```python
from build123d import *

# Parameters (mm, degrees)
SKETCH_1_R      = 3.4
SKETCH_1_W      = 10.3
SKETCH_1_H      = 10.3
EXTRUDE_1_DEPTH = 100


with BuildPart() as part:
    # 草图1 → 凸台-拉伸1 (new body)
    with BuildSketch(Plane.XY):
        with BuildLine():
            Line((-22.463172707, 9.357012623), (-25.363172707, 9.357012623))
            Line((-25.363172707, 9.357012623), (-25.363172707, 17.757012623))
            Line((-25.363172707, 17.757012623), (-22.963172707, 17.757012623))
            ThreePointArc((-22.963172707, 17.757012623), (-22.609619316, 17.903459232), (-22.463172707, 18.257012623))
            Line((-22.463172707, 18.257012623), (-22.463172707, 20.257012623))
            ThreePointArc((-22.463172707, 20.257012623), (-22.609619316, 20.610566013), (-22.963172707, 20.757012623))
            Line((-22.963172707, 20.757012623), (-37.863172707, 20.757012623))
            ThreePointArc((-37.863172707, 20.757012623), (-38.216726098, 20.610566013), (-38.363172707, 20.257012623))
            Line((-38.363172707, 20.257012623), (-38.363172707, 5.357012623))
            ThreePointArc((-38.363172707, 5.357012623), (-38.216726098, 5.003459232), (-37.863172707, 4.857012623))
            Line((-37.863172707, 4.857012623), (-35.863172707, 4.857012623))
            ThreePointArc((-35.863172707, 4.857012623), (-35.509619316, 5.003459232), (-35.363172707, 5.357012623))
            Line((-35.363172707, 5.357012623), (-35.363172707, 7.757012623))
            Line((-35.363172707, 7.757012623), (-26.963172707, 7.757012623))
            Line((-26.963172707, 7.757012623), (-26.963172707, 4.857012623))
            Line((-26.963172707, 4.857012623), (-25.420279488, 6.399905842))
            Line((-25.420279488, 6.399905842), (-23.217718457, 4.19734481))
            ThreePointArc((-23.217718457, 4.19734481), (-24.313172707, 0.757012623), (-23.217718457, -2.683319565))
            Line((-23.217718457, -2.683319565), (-25.420279488, -4.885880596))
            Line((-25.420279488, -4.885880596), (-26.963172707, -3.342987377))
            Line((-26.963172707, -3.342987377), (-26.963172707, -6.242987377))
            Line((-26.963172707, -6.242987377), (-35.363172707, -6.242987377))
            Line((-35.363172707, -6.242987377), (-35.363172707, -3.842987377))
            ThreePointArc((-35.363172707, -3.842987377), (-35.509619316, -3.489433987), (-35.863172707, -3.342987377))
            Line((-35.863172707, -3.342987377), (-37.863172707, -3.342987377))
            ThreePointArc((-37.863172707, -3.342987377), (-38.216726098, -3.489433987), (-38.363172707, -3.842987377))
            Line((-38.363172707, -3.842987377), (-38.363172707, -18.742987377))
            ThreePointArc((-38.363172707, -18.742987377), (-38.216726098, -19.096540768), (-37.863172707, -19.242987377))
            Line((-37.863172707, -19.242987377), (-22.963172707, -19.242987377))
            ThreePointArc((-22.963172707, -19.242987377), (-22.609619316, -19.096540768), (-22.463172707, -18.742987377))
            Line((-22.463172707, -18.742987377), (-22.463172707, -16.742987377))
            ThreePointArc((-22.463172707, -16.742987377), (-22.609619316, -16.389433987), (-22.963172707, -16.242987377))
            Line((-22.963172707, -16.242987377), (-25.363172707, -16.242987377))
            Line((-25.363172707, -16.242987377), (-25.363172707, -7.842987377))
            Line((-25.363172707, -7.842987377), (-22.463172707, -7.842987377))
            Line((-22.463172707, -7.842987377), (-24.006065926, -6.300094158))
            Line((-24.006065926, -6.300094158), (-21.803504895, -4.097533127))
            ThreePointArc((-21.803504895, -4.097533127), (-18.363172707, -5.192987377), (-14.922840519, -4.097533127))
            Line((-14.922840519, -4.097533127), (-12.720279488, -6.300094158))
            Line((-12.720279488, -6.300094158), (-14.263172707, -7.842987377))
            Line((-14.263172707, -7.842987377), (-11.363172707, -7.842987377))
            Line((-11.363172707, -7.842987377), (-11.363172707, -16.242987377))
            Line((-11.363172707, -16.242987377), (-13.763172707, -16.242987377))
            ThreePointArc((-13.763172707, -16.242987377), (-14.116726098, -16.389433987), (-14.263172707, -16.742987377))
            Line((-14.263172707, -16.742987377), (-14.263172707, -18.742987377))
            ThreePointArc((-14.263172707, -18.742987377), (-14.116726098, -19.096540768), (-13.763172707, -19.242987377))
            Line((-13.763172707, -19.242987377), (1.136827293, -19.242987377))
            Line((1.136827293, -19.242987377), (2.136827293, -19.242987377))
            Line((2.136827293, -19.242987377), (17.036827293, -19.242987377))
            ThreePointArc((17.036827293, -19.242987377), (17.390380684, -19.096540768), (17.536827293, -18.742987377))
            Line((17.536827293, -18.742987377), (17.536827293, -16.742987377))
            ThreePointArc((17.536827293, -16.742987377), (17.390380684, -16.389433987), (17.036827293, -16.242987377))
            Line((17.036827293, -16.242987377), (14.636827293, -16.242987377))
            Line((14.636827293, -16.242987377), (14.636827293, -7.842987377))
            Line((14.636827293, -7.842987377), (17.536827293, -7.842987377))
            Line((17.536827293, -7.842987377), (15.993934074, -6.300094158))
            Line((15.993934074, -6.300094158), (18.196495105, -4.097533127))
            ThreePointArc((18.196495105, -4.097533127), (21.636827293, -5.192987377), (25.077159481, -4.097533127))
            Line((25.077159481, -4.097533127), (27.279720512, -6.300094158))
            Line((27.279720512, -6.300094158), (25.736827293, -7.842987377))
            Line((25.736827293, -7.842987377), (28.636827293, -7.842987377))
            Line((28.636827293, -7.842987377), (28.636827293, -16.242987377))
            Line((28.636827293, -16.242987377), (26.236827293, -16.242987377))
            ThreePointArc((26.236827293, -16.242987377), (25.883273902, -16.389433987), (25.736827293, -16.742987377))
            Line((25.736827293, -16.742987377), (25.736827293, -18.742987377))
            ThreePointArc((25.736827293, -18.742987377), (25.883273902, -19.096540768), (26.236827293, -19.242987377))
            Line((26.236827293, -19.242987377), (41.136827293, -19.242987377))
            ThreePointArc((41.136827293, -19.242987377), (41.490380684, -19.096540768), (41.636827293, -18.742987377))
            Line((41.636827293, -18.742987377), (41.636827293, -3.842987377))
            ThreePointArc((41.636827293, -3.842987377), (41.490380684, -3.489433987), (41.136827293, -3.342987377))
            Line((41.136827293, -3.342987377), (39.136827293, -3.342987377))
            ThreePointArc((39.136827293, -3.342987377), (38.783273902, -3.489433987), (38.636827293, -3.842987377))
            Line((38.636827293, -3.842987377), (38.636827293, -6.242987377))
            Line((38.636827293, -6.242987377), (30.236827293, -6.242987377))
            Line((30.236827293, -6.242987377), (30.236827293, -3.342987377))
            Line((30.236827293, -3.342987377), (28.693934074, -4.885880596))
            Line((28.693934074, -4.885880596), (26.491373043, -2.683319565))
            ThreePointArc((26.491373043, -2.683319565), (27.586827293, 0.757012623), (26.491373043, 4.19734481))
            Line((26.491373043, 4.19734481), (28.693934074, 6.399905842))
            Line((28.693934074, 6.399905842), (30.236827293, 4.857012623))
            Line((30.236827293, 4.857012623), (30.236827293, 7.757012623))
            Line((30.236827293, 7.757012623), (38.636827293, 7.757012623))
            Line((38.636827293, 7.757012623), (38.636827293, 5.357012623))
            ThreePointArc((38.636827293, 5.357012623), (38.783273902, 5.003459232), (39.136827293, 4.857012623))
            Line((39.136827293, 4.857012623), (41.136827293, 4.857012623))
            ThreePointArc((41.136827293, 4.857012623), (41.490380684, 5.003459232), (41.636827293, 5.357012623))
            Line((41.636827293, 5.357012623), (41.636827293, 20.257012623))
            ThreePointArc((41.636827293, 20.257012623), (41.490380684, 20.610566013), (41.136827293, 20.757012623))
            Line((41.136827293, 20.757012623), (26.236827293, 20.757012623))
            ThreePointArc((26.236827293, 20.757012623), (25.883273902, 20.610566013), (25.736827293, 20.257012623))
            Line((25.736827293, 20.257012623), (25.736827293, 18.257012623))
            ThreePointArc((25.736827293, 18.257012623), (25.883273902, 17.903459232), (26.236827293, 17.757012623))
            Line((26.236827293, 17.757012623), (28.636827293, 17.757012623))
            Line((28.636827293, 17.757012623), (28.636827293, 9.357012623))
            Line((28.636827293, 9.357012623), (25.736827293, 9.357012623))
            Line((25.736827293, 9.357012623), (27.279720512, 7.814119404))
            Line((27.279720512, 7.814119404), (25.077159481, 5.611558373))
            ThreePointArc((25.077159481, 5.611558373), (21.636827293, 6.707012623), (18.196495105, 5.611558373))
            Line((18.196495105, 5.611558373), (15.993934074, 7.814119404))
            Line((15.993934074, 7.814119404), (17.536827293, 9.357012623))
            Line((17.536827293, 9.357012623), (14.636827293, 9.357012623))
            Line((14.636827293, 9.357012623), (14.636827293, 17.757012623))
            Line((14.636827293, 17.757012623), (17.036827293, 17.757012623))
            ThreePointArc((17.036827293, 17.757012623), (17.390380684, 17.903459232), (17.536827293, 18.257012623))
            Line((17.536827293, 18.257012623), (17.536827293, 20.257012623))
            ThreePointArc((17.536827293, 20.257012623), (17.390380684, 20.610566013), (17.036827293, 20.757012623))
            Line((17.036827293, 20.757012623), (2.136827293, 20.757012623))
            Line((2.136827293, 20.757012623), (1.136827293, 20.757012623))
            Line((1.136827293, 20.757012623), (-13.763172707, 20.757012623))
            ThreePointArc((-13.763172707, 20.757012623), (-14.116726098, 20.610566013), (-14.263172707, 20.257012623))
            Line((-14.263172707, 20.257012623), (-14.263172707, 18.257012623))
            ThreePointArc((-14.263172707, 18.257012623), (-14.116726098, 17.903459232), (-13.763172707, 17.757012623))
            Line((-13.763172707, 17.757012623), (-11.363172707, 17.757012623))
            Line((-11.363172707, 17.757012623), (-11.363172707, 9.357012623))
            Line((-11.363172707, 9.357012623), (-14.263172707, 9.357012623))
            Line((-14.263172707, 9.357012623), (-12.720279488, 7.814119404))
            Line((-12.720279488, 7.814119404), (-14.922840519, 5.611558373))
            ThreePointArc((-14.922840519, 5.611558373), (-18.363172707, 6.707012623), (-21.803504895, 5.611558373))
            Line((-21.803504895, 5.611558373), (-24.006065926, 7.814119404))
            Line((-24.006065926, 7.814119404), (-22.463172707, 9.357012623))
        make_face()
        with Locations((-18.363172707, 0.757012623)):
            Circle(SKETCH_1_R, mode=Mode.SUBTRACT)
        with Locations((21.636827293, 0.757012623)):
            Circle(SKETCH_1_R, mode=Mode.SUBTRACT)
        with Locations((-31.513172707, 13.907012623)):
            Rectangle(SKETCH_1_W, SKETCH_1_H, mode=Mode.SUBTRACT)
        with BuildLine():
            Line((-9.363172707, 17.757012623), (-9.363172707, 8.34279906))
            Line((-9.363172707, 8.34279906), (-13.508626957, 4.19734481))
            ThreePointArc((-13.508626957, 4.19734481), (-12.413172707, 0.757012623), (-13.508626957, -2.683319565))
            Line((-13.508626957, -2.683319565), (-9.363172707, -6.828773815))
            Line((-9.363172707, -6.828773815), (-9.363172707, -16.242987377))
            ThreePointArc((-9.363172707, -16.242987377), (-9.070279488, -16.950094158), (-8.363172707, -17.242987377))
            Line((-8.363172707, -17.242987377), (11.636827293, -17.242987377))
            ThreePointArc((11.636827293, -17.242987377), (12.343934074, -16.950094158), (12.636827293, -16.242987377))
            Line((12.636827293, -16.242987377), (12.636827293, -6.828773815))
            Line((12.636827293, -6.828773815), (16.782281543, -2.683319565))
            ThreePointArc((16.782281543, -2.683319565), (15.686827293, 0.757012623), (16.782281543, 4.19734481))
            Line((16.782281543, 4.19734481), (12.636827293, 8.34279906))
            Line((12.636827293, 8.34279906), (12.636827293, 17.757012623))
            ThreePointArc((12.636827293, 17.757012623), (12.343934074, 18.464119404), (11.636827293, 18.757012623))
            Line((11.636827293, 18.757012623), (-8.363172707, 18.757012623))
            ThreePointArc((-8.363172707, 18.757012623), (-9.070279488, 18.464119404), (-9.363172707, 17.757012623))
        make_face(mode=Mode.SUBTRACT)
        with Locations((-31.513172707, -12.392987377)):
            Rectangle(SKETCH_1_W, SKETCH_1_H, mode=Mode.SUBTRACT)
        with Locations((34.786827293, 13.907012623)):
            Rectangle(SKETCH_1_W, SKETCH_1_H, mode=Mode.SUBTRACT)
        with Locations((34.786827293, -12.392987377)):
            Rectangle(SKETCH_1_W, SKETCH_1_H, mode=Mode.SUBTRACT)
    extrude(amount=EXTRUDE_1_DEPTH)


solid = part.part
```
Work out the finished part from the listing and answer in its coordinate system (mm). Coordinates: 2 decimals unless noted, no trailing zeros. Loops run counter-clockwise (first coordinate to the right, second up) from the corner with the lowest first, then second, coordinate; pieces in that order, holes last. Notation, with made-up numbers: M 66.5,-35 L 84.5,-35 A10 ccw 84.5,-20 Z; hole C -7,-14.5 d6. An arc over 180 degrees is marked long. Use CSV: the item, a comma, the result in double quotes. Start each with the question number.
(1) Find section D-D, the plane z = 39. State how many separate pieces and enclosed holes the cut face has, then the cut area to 3 significant figures.
(2) Consider line 1 (Y direction, x = -30, z = 21.5); line 2 (X direction, y = -9, z = 10); line 3 (Y direction, x = 15, z = 40). Determine where each line is inside the solid, lowest interval first.
(3) Given pin 1 Ø1.5 at (y, z) = (2.5, 49) entering from +X, flat-ended and moving along its own axis, determine where the tip first touches the part or whether it passes through.
(4) Find section B-B, the plane y = 13.5. Give the vertices of the cut face in (x, z), then the cut area to 3 significant figures.
(5) Find section A-A, the plane x = -31. Give the vertices of the cut face in (y, z), then the cut area to 3 significant figures.
(6) For a pull along Y with two mould halves and no side action, classify faces 1 (the face through (38.637, 7, 49)), 2 (the face through (34, 20.757, 49)) as +Y half, -Y half, draft (parallel to the pull), parting line (faces both ways), or undercut.
(7) Find section C-C, the plane x = 8.5. Give the vertices of the cut face in (y, z).
Recorded:
1,separate pieces,"1"
1,enclosed holes,"7"
1,area,"797 mm^2"
2,line 1,"y = -19.24 to -17.54, -7.24 to -6.24, 7.76 to 8.76, 19.06 to 20.76"
2,line 2,"x = -38.36 to -36.66, -26.36 to -25.36, -11.36 to -9.36, 12.64 to 14.64, 28.64 to 29.64, 39.94 to 41.64"
2,line 3,"y = -19.24 to -16.24, -7.84 to -4.47, 5.98 to 9.36, 17.76 to 20.76"
3,pin 1,"stops at x = 27.5"
4,outline,"M -38.36,0 L -36.66,0 L -36.66,100 L -38.36,100 Z; M -26.36,0 L -25.36,0 L -25.36,100 L -26.36,100 Z; M -11.36,0 L -9.36,0 L -9.36,100 L -11.36,100 Z; M 12.64,0 L 14.64,0 L 14.64,100 L 12.64,100 Z; M 28.64,0 L 29.64,0 L 29.64,100 L 28.64,100 Z; M 39.94,0 L 41.64,0 L 41.64,100 L 39.94,100 Z"
4,area,"940 mm^2"
5,outline,"M -19.24,0 L -17.54,0 L -17.54,100 L -19.24,100 Z; M -7.24,0 L -6.24,0 L -6.24,100 L -7.24,100 Z; M 7.76,0 L 8.76,0 L 8.76,100 L 7.76,100 Z; M 19.06,0 L 20.76,0 L 20.76,100 L 19.06,100 Z"
5,area,"540 mm^2"
6,face 1,"undercut"
6,face 2,"+Y half"
7,outline,"M -19.24,0 L -17.24,0 L -17.24,100 L -19.24,100 Z; M 18.76,0 L 20.76,0 L 20.76,100 L 18.76,100 Z"
